```python
from build123d import *

# Parameters (mm, degrees)
SKETCH1_R                  = 43
SKETCH1_R_2                = 30.5
BOSS_EXTRUDE1_DEPTH        = 1.5875
SKETCH2_R                  = 1.25
SKETCH2_R_2                = 1.477643217
CUT_EXTRUDE1_DEPTH         = 2.5875
M2_5_CLEARANCE_HOLE1_D     = 2.9
M2_5_CLEARANCE_HOLE1_DEPTH = 6
M2_5_CLEARANCE_HOLE1_TIP   = 0.871247898
CUT_EXTRUDE2_DEPTH         = 2.5875


with BuildPart() as part:
    # Sketch1 → Boss-Extrude1 (new body)
    with BuildSketch(Plane(origin=(0, 0, 0), x_dir=(0, 0, -1), z_dir=(1, 0, 0))):
        Circle(SKETCH1_R)
        Circle(SKETCH1_R_2, mode=Mode.SUBTRACT)
    extrude(amount=BOSS_EXTRUDE1_DEPTH)

    # Sketch2 → Cut-Extrude1 (cut, through all)
    with BuildSketch(Plane(origin=(1.5875, 0, 0), x_dir=(0, 0, -1), z_dir=(1, 0, 0))):
        with Locations((0, 40)):
            Circle(SKETCH2_R)
        with Locations((4.181138531, 39.780875815)):
            Circle(SKETCH2_R)
        with Locations((8.316467633, 39.125904029)):
            Circle(SKETCH2_R)
        with Locations((12.360679775, 38.042260652)):
            Circle(SKETCH2_R)
        with Locations((16.269465723, 36.541818306)):
            Circle(SKETCH2_R)
        with Locations((20, 34.641016151)):
            Circle(SKETCH2_R)
        with Locations((23.511410092, 32.360679775)):
            Circle(SKETCH2_R)
        with Locations((26.765224254, 29.725793019)):
            Circle(SKETCH2_R)
        with Locations((29.725793019, 26.765224254)):
            Circle(SKETCH2_R)
        with Locations((32.360679775, 23.511410092)):
            Circle(SKETCH2_R)
        with Locations((34.641016151, 20)):
            Circle(SKETCH2_R)
        with Locations((36.541818306, 16.269465723)):
            Circle(SKETCH2_R)
        with Locations((38.042260652, 12.360679775)):
            Circle(SKETCH2_R)
        with Locations((39.125904029, 8.316467633)):
            Circle(SKETCH2_R)
        with Locations((39.780875815, 4.181138531)):
            Circle(SKETCH2_R)
        with Locations((40, 0)):
            Circle(SKETCH2_R)
        with Locations((39.780875815, -4.181138531)):
            Circle(SKETCH2_R)
        with Locations((39.125904029, -8.316467633)):
            Circle(SKETCH2_R)
        with Locations((38.042260652, -12.360679775)):
            Circle(SKETCH2_R)
        with Locations((36.541818306, -16.269465723)):
            Circle(SKETCH2_R)
        with Locations((34.641016151, -20)):
            Circle(SKETCH2_R)
        with Locations((32.360679775, -23.511410092)):
            Circle(SKETCH2_R)
        with Locations((29.725793019, -26.765224254)):
            Circle(SKETCH2_R)
        with Locations((26.765224254, -29.725793019)):
            Circle(SKETCH2_R)
        with Locations((23.511410092, -32.360679775)):
            Circle(SKETCH2_R)
        with Locations((20, -34.641016151)):
            Circle(SKETCH2_R)
        with Locations((16.269465723, -36.541818306)):
            Circle(SKETCH2_R)
        with Locations((12.360679775, -38.042260652)):
            Circle(SKETCH2_R)
        with Locations((8.316467633, -39.125904029)):
            Circle(SKETCH2_R)
        with Locations((4.181138531, -39.780875815)):
            Circle(SKETCH2_R)
        with Locations((0, -40)):
            Circle(SKETCH2_R)
        with Locations((-4.181138531, -39.780875815)):
            Circle(SKETCH2_R)
        with Locations((-8.316467633, -39.125904029)):
            Circle(SKETCH2_R)
        with Locations((-12.360679775, -38.042260652)):
            Circle(SKETCH2_R)
        with Locations((-16.269465723, -36.541818306)):
            Circle(SKETCH2_R)
        with Locations((-20, -34.641016151)):
            Circle(SKETCH2_R)
        with Locations((-23.511410092, -32.360679775)):
            Circle(SKETCH2_R)
        with Locations((-26.765224254, -29.725793019)):
            Circle(SKETCH2_R)
        with Locations((-29.725793019, -26.765224254)):
            Circle(SKETCH2_R)
        with Locations((-32.360679775, -23.511410092)):
            Circle(SKETCH2_R)
        with Locations((-34.641016151, -20)):
            Circle(SKETCH2_R)
        with Locations((-36.541818306, -16.269465723)):
            Circle(SKETCH2_R)
        with Locations((-38.042260652, -12.360679775)):
            Circle(SKETCH2_R)
        with Locations((-39.125904029, -8.316467633)):
            Circle(SKETCH2_R)
        with Locations((-39.780875815, -4.181138531)):
            Circle(SKETCH2_R)
        with Locations((-40, 0)):
            Circle(SKETCH2_R)
        with Locations((-39.780875815, 4.181138531)):
            Circle(SKETCH2_R)
        with Locations((-39.125904029, 8.316467633)):
            Circle(SKETCH2_R)
        with Locations((-38.042260652, 12.360679775)):
            Circle(SKETCH2_R)
        with Locations((-36.541818306, 16.269465723)):
            Circle(SKETCH2_R)
        with Locations((-34.641016151, 20)):
            Circle(SKETCH2_R)
        with Locations((-32.360679775, 23.511410092)):
            Circle(SKETCH2_R)
        with Locations((-29.725793019, 26.765224254)):
            Circle(SKETCH2_R)
        with Locations((-26.765224254, 29.725793019)):
            Circle(SKETCH2_R)
        with Locations((-23.511410092, 32.360679775)):
            Circle(SKETCH2_R)
        with Locations((-20, 34.641016151)):
            Circle(SKETCH2_R)
        with Locations((-16.269465723, 36.541818306)):
            Circle(SKETCH2_R)
        with Locations((-12.360679775, 38.042260652)):
            Circle(SKETCH2_R)
        with Locations((-8.316467633, 39.125904029)):
            Circle(SKETCH2_R)
        with Locations((-4.181138531, 39.780875815)):
            Circle(SKETCH2_R)
        with Locations((-29.444863729, 17)):
            Circle(SKETCH2_R_2)
    extrude(amount=-CUT_EXTRUDE1_DEPTH, mode=Mode.SUBTRACT)

    # M2.5 Clearance Hole1
    with Locations(Plane(origin=(1.5875, 0, 0), x_dir=(0, 0, -1), z_dir=(1, 0, 0))):
        with Locations((0, 34), (-34, 0), (34, 0), (0, -34)):
            Hole(M2_5_CLEARANCE_HOLE1_D / 2, depth=M2_5_CLEARANCE_HOLE1_DEPTH)
            with Locations((0, 0, -(M2_5_CLEARANCE_HOLE1_DEPTH + M2_5_CLEARANCE_HOLE1_TIP / 2))):  # 118° drill point
                Cone(0, M2_5_CLEARANCE_HOLE1_D / 2, M2_5_CLEARANCE_HOLE1_TIP, mode=Mode.SUBTRACT)

    # Sketch6 → Cut-Extrude2 (cut, through all)
    with BuildSketch(Plane(origin=(1.5875, 0, 0), x_dir=(0, 0, -1), z_dir=(1, 0, 0))):
        with BuildLine():
            Line((28.828838325, -16.066987298), (31.859927238, -17.816987298))
            ThreePointArc((31.859927238, -17.816987298), (32.04293994, -18.5), (31.359927238, -18.683012702))
            Line((31.359927238, -18.683012702), (28.328838325, -16.933012702))
            ThreePointArc((28.328838325, -16.933012702), (28.145825623, -16.25), (28.828838325, -16.066987298))
        make_face()
    extrude(amount=-CUT_EXTRUDE2_DEPTH, mode=Mode.SUBTRACT)


solid = part.part
```
Input: part model. Units: mm. Frame: model coordinates. Round coordinates to 2 decimals unless told otherwise and drop trailing zeros. Order: outer loops, then holes, each group sorted by start corner. A loop starts at its lowest first (then second) coordinate and runs counter-clockwise, first axis right, second up. Notation, with made-up numbers: (10.5, 10) - (35.5, 10) arc R17 ccw to (35.5, 21) - close; hole circle Ø9 at (-38, 43.25). An arc over 180 degrees is marked (long way). Answer in a Markdown table with one row per item.
Item 1: Pin query (flat end, axial travel): pin 1 (2 mm diameter, centred on y = -16.27, z = -36.54, fed in from +X). Return the tip coordinate at first contact, or that it passes through.
Model answer:
| item | result |
|---|---|
| pin 1 | passes through |
Item 2: Section query A-A (y = 0). Return the cut outline in (x, z).
Model answer:
| item | result |
|---|---|
| outline | (0, -43) - (1.59, -43) - (1.59, -41.25) - (0, -41.25) - close; (0, -38.75) - (1.59, -38.75) - (1.59, -35.45) - (0, -35.45) - close; (0, -32.55) - (1.59, -32.55) - (1.59, -30.5) - (0, -30.5) - close; (0, 30.5) - (1.59, 30.5) - (1.59, 32.55) - (0, 32.55) - close; (0, 35.45) - (1.59, 35.45) - (1.59, 38.75) - (0, 38.75) - close; (0, 41.25) - (1.59, 41.25) - (1.59, 43) - (0, 43) - close |
Item 3: Mould query, pull axis Z, two halves, no side actions, for faces 1 (the flat face through (0, 29.3, -9)), 2 (the cylindrical face through (0.805, -19.945, -33.392)). Classes: released by +Z, released by -Z, zero draft, split by the parting line, or undercut.
Model answer:
| item | result |
|---|---|
| face 1 | zero draft |
| face 2 | undercut |
Item 4: Line query: line 1 (Z direction, x = 0.25, y = 35.5); line 2 (Y direction, x = 1.05, z = -34.5). Output: solid intervals per line, ascending.
Model answer:
| item | result |
|---|---|
| line 1 | z = -24.26 to -20.91, -19.09 to -16.96, -15.58 to 15.58, 16.96 to 19.09, 20.91 to 24.26 |
| line 2 | y = -25.67 to -21.24, -18.76 to -1.36, 1.36 to 18.76, 21.24 to 25.67 |
Item 5: Section query C-C (z = -20). Return the cut outline in (x, y).
Model answer:
| item | result |
|---|---|
| outline | (0, -38.07) - (1.59, -38.07) - (1.59, -35.89) - (0, -35.89) - close; (0, -33.39) - (1.59, -33.39) - (1.59, -23.03) - (0, -23.03) - close; (0, 23.03) - (1.59, 23.03) - (1.59, 33.39) - (0, 33.39) - close; (0, 35.89) - (1.59, 35.89) - (1.59, 38.07) - (0, 38.07) - close |
